Design review of the part shown in the three views and the two pictorial views. Dimensions are in mm from the part's minimum x, y and z. Coordinates: 2 decimals unless noted, no trailing zeros. Loops run counter-clockwise (first coordinate to the right, second up) from the corner with the lowest first, then second, coordinate; pieces in that order, holes last.
Q1. For P1, Ø0.9, axis at x = 6.5, y = 1.5, coming from the +Z side; P2, Ø6, axis at x = 21.5, z = 31.5, coming from the -Y side; P3, Ø1.5, axis at y = 1.5, z = 45, coming from the -X side, all flat-tipped, find the tip position at first contact; note any pin that passes through.
Q2. Add section B-B on z = 44. Give the boundary of the cut face in (x, y).
Q3. Wall thickness on probe 1 along Z at (x, y) = (8, 0.4); probe 2 along X at (y, z) = (1, 46.5): over which ranges is each line inside the solid? List them lowest first.
Q4. Add section A-A on y = 0.45. Give the boundary of the cut face in (x, z).
Q5. Add section C-C on x = 3.5. Give the boundary of the cut face in (y, z), and give its area (4 significant figures).
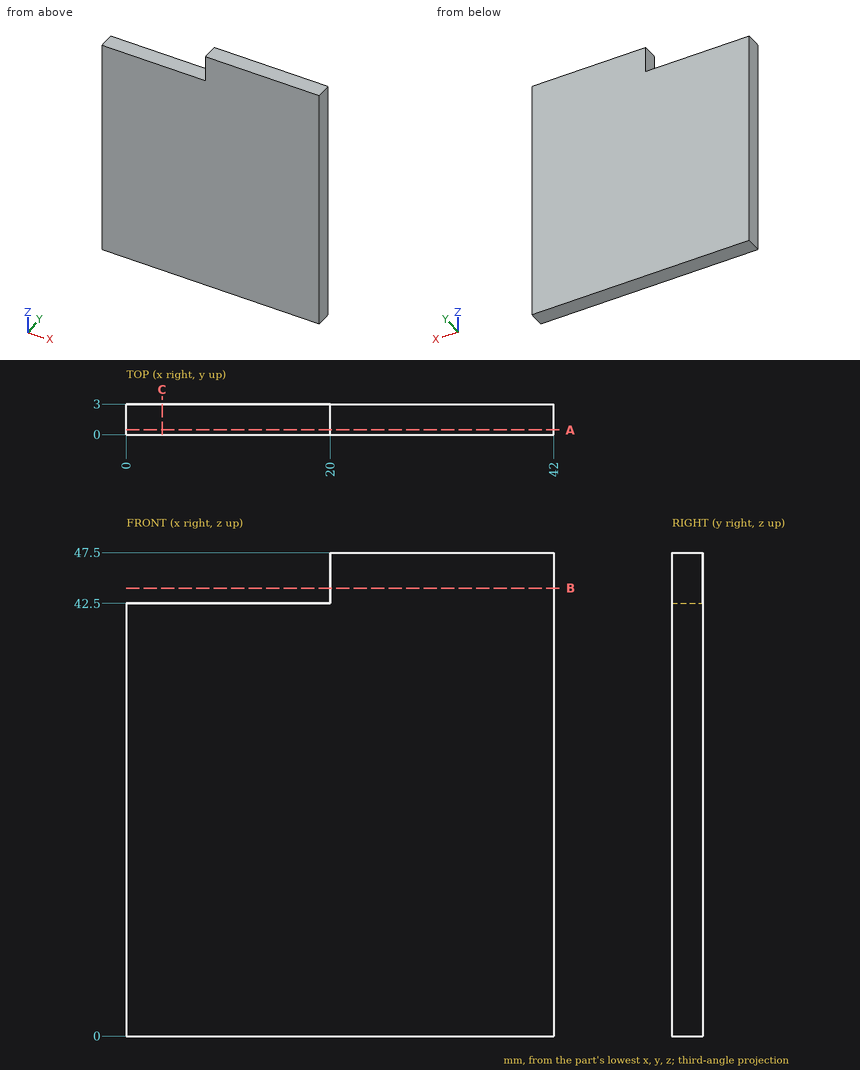
Entries:
1. P1: stops at z = 42.5
1. P2: stops at y = 0
1. P3: stops at x = 20
2. outline: (20, 0) - (42, 0) - (42, 3) - (20, 3) - close
3. probe 1: z = 0 to 42.5
3. probe 2: x = 20 to 42
4. outline: (0, 0) - (42, 0) - (42, 47.5) - (20, 47.5) - (20, 42.5) - (0, 42.5) - close
5. outline: (0, 0) - (3, 0) - (3, 42.5) - (0, 42.5) - close
5. area: 127.5 mm2
